Geometry: see drawing. Coordinates: mm, zero at the bounding-box minimum. A direction names the side the tool comes from. Coordinates: 2 decimals unless noted, no trailing zeros. Order: outer loops, then holes, each group sorted by start corner. A loop starts at its lowest first (then second) coordinate and runs counter-clockwise, first axis right, second up. Notation, with made-up numbers: (32.5, -21) -> (69.5, -21) arc R15 cw to (69.5, -13) -> close; hole circle Ø1 at (-20, 64). An arc over 180 degrees is marked (long way). Write each question's results on one line, items separated by ' | '.
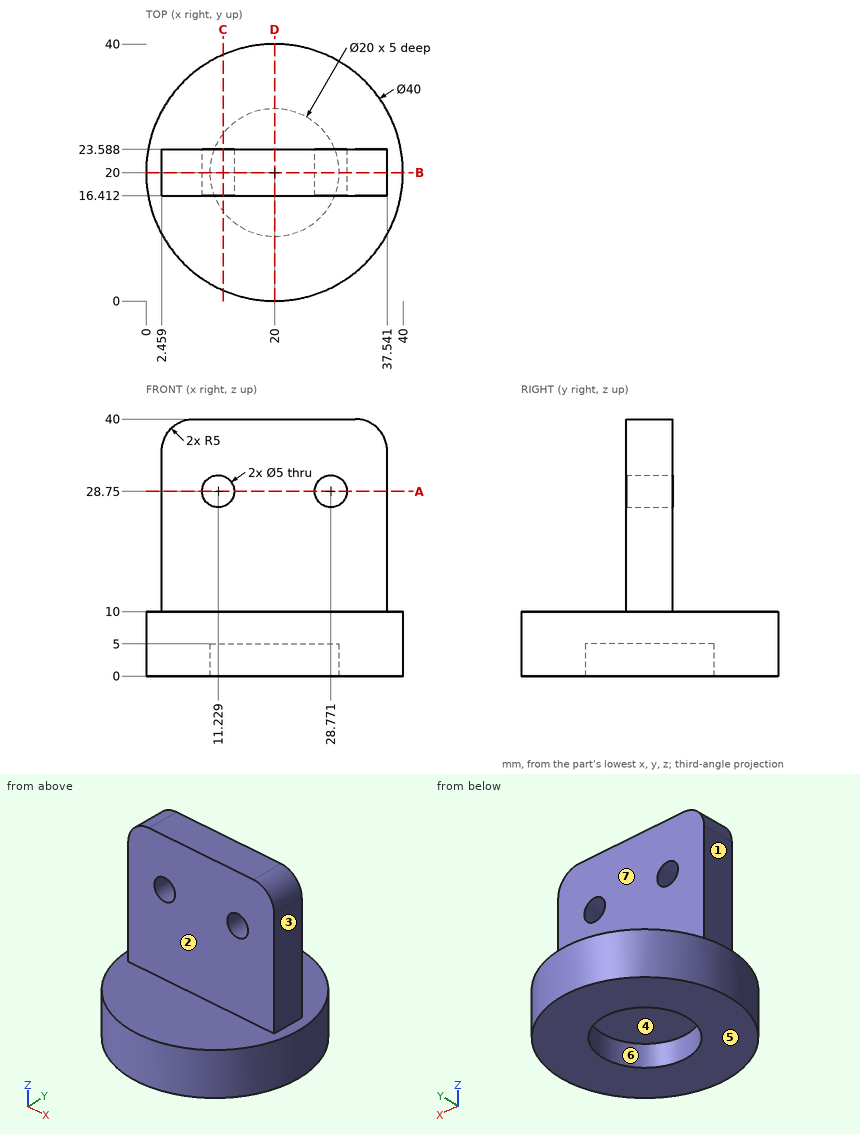
(1) Cut plane A-A, the plane z = 28.75. Return loops of the section in (x, y), plus the area to 3 significant figures.
Return value:
outline: (2.46, 16.41) -> (8.73, 16.41) -> (8.73, 23.59) -> (2.46, 23.59) -> close; (13.73, 16.41) -> (26.27, 16.41) -> (26.27, 23.59) -> (13.73, 23.59) -> close; (31.27, 16.41) -> (37.54, 16.41) -> (37.54, 23.59) -> (31.27, 23.59) -> close | area: 180 mm2
(2) Line query: line 1 along X through (y, z) = (20.25, 28.75); line 2 along Y through (x, z) = (20, 1.65); line 3 along Y through (x, z) = (26, 38). Output: solid intervals per line, ascending. Write a range as from..to.
Return value:
line 1: 2.46..8.73, 13.73..26.27, 31.27..37.54 | line 2: 0..10, 30..40 | line 3: 16.41..23.59
(3) Mould query, pull axis Y, two halves, no side actions, for the marked faces 5, 6 and 7. Classes: +Y half, -Y half, draft (parallel to the pull), parting line (faces both ways), or undercut.
Return value:
face 5: draft | face 6: undercut | face 7: +Y half
(4) Cut plane D-D, the plane x = 20. Return loops of the section in (y, z).
Return value:
outline: (0, 0) -> (10, 0) -> (10, 5) -> (30, 5) -> (30, 0) -> (40, 0) -> (40, 10) -> (23.59, 10) -> (23.59, 40) -> (16.41, 40) -> (16.41, 10) -> (0, 10) -> close
(5) Cut plane B-B, the plane y = 20. Return loops of the section in (x, z).
Return value:
outline: (0, 0) -> (10, 0) -> (10, 5) -> (30, 5) -> (30, 0) -> (40, 0) -> (40, 10) -> (37.54, 10) -> (37.54, 35) arc R5 ccw to (32.54, 40) -> (7.46, 40) arc R5 ccw to (2.46, 35) -> (2.46, 10) -> (0, 10) -> close; hole circle Ø5 at (11.23, 28.75); hole circle Ø5 at (28.77, 28.75)
(6) Reachability of the marked faces 1, 2, 3 and 4 from +Z, -Z, +X, -X, +Y, -Y: full face, straight path, thin tool, end or side. Return the list, or none.
Return value:
face 1: +Z, -X, +Y, -Y | face 2: +Z, +X, -X, -Y | face 3: +Z, +X, +Y, -Y | face 4: -Z
(7) Cut plane C-C, the plane x = 12. Return loops of the section in (y, z).
Return value:
outline: (1.67, 0) -> (14, 0) -> (14, 5) -> (26, 5) -> (26, 0) -> (38.33, 0) -> (38.33, 10) -> (23.59, 10) -> (23.59, 26.37) -> (16.41, 26.37) -> (16.41, 10) -> (1.67, 10) -> close; (16.41, 31.13) -> (23.59, 31.13) -> (23.59, 40) -> (16.41, 40) -> close
(8) Pin query (flat end, axial travel): P1, Ø3.5, axis at y = 20, z = 22.5, coming from the +X side; P2, Ø8, axis at x = 11.23, z = 28.75, coming from the +Y side; P3, Ø6, axis at x = 28.77, z = 28.75, coming from the -Y side. Return the tip coordinate at first contact, or that it passes through.
Return value:
P1: x = 37.54 | P2: y = 23.59 | P3: y = 16.41
